Can you work these out from the model? Positions are in its coordinate system, mm. A direction names the side the tool comes from. Give positions to 0.01 mm unless a question says otherwise; leave off trailing zeros. Order: outer loops, then holes, each group sorted by start corner. A loop starts at its lowest first (then second) coordinate and runs counter-clockwise, first axis right, second up. Notation, with made-up numbers: (-35, 88.5) - (24, 88.5) arc R7 ccw to (24, 96.5) - close; hole circle Ø1 at (56, 83). An arc over 180 degrees is marked (long way). One line per question, with ' | ' between items.
Autodesk Inventor part; units mm, degrees
ref_plane "Work Plane1" through (4.68, 0, 0) normal (0, -0.866, 0.5) x (-1, 0, 0)
ref_plane "YZ Plane" through (0, 0, 0) normal (1, 0, 0) x (0, 1, 0)
ref_plane "XZ Plane" through (0, 0, 0) normal (0, 1, 0) x (-1, 0, 0)
sketch "Sketch1" plane through (0, 0, 0) normal (1, 0, 0) x (0, 1, 0)
  line L0 (-9.815, 0) -> (-4.9075, 8.5)
  line L1 (-4.9075, 8.5) -> (4.9075, 8.5)
  line L2 (4.9075, 8.5) -> (9.815, 0)
  line L3 (9.815, 0) -> (4.9075, -8.5)
  line L4 (4.9075, -8.5) -> (-4.9075, -8.5)
  line L5 (-4.9075, -8.5) -> (-9.815, 0)
  point P0 (0, 0)
  point P1 (0, 0)
  dimension "d0" = 19.6299
extrude "Body" add sketch "Sketch1" along normal blind 7.8
sketch "Sketch2" plane through (0, 0, 0) normal (0, 0, 1) x (1, 0, 0)
  line L0 (7.8, 8.5) -> (10.5, 8.5)
  line L1 (10.5, 8.5) -> (10.5, 5.8)
  line L2 (10.5, 5.8) -> (12.3, 5.8)
  arc A0 (18.1, 0) -> (12.3, 5.8) centre (12.3, 0) ccw
  line L3 (-3.8602, 0) -> (23.1615, 0)
  line L4 (0, -7.589) -> (0, 11.1815)
  line L5 (7.8, 0) -> (18.1, 0)
  line L6 (7.8, -4.9075) -> (7.8, 4.9075)
  line L7 (7.8, 0) -> (7.8, 8.5)
  point P0 (0, 0)
  dimension "d8" = 5.8
  dimension "d9" = 17
  dimension "d10" = 18.1
  dimension "d11" = 10.5
  dimension "d12" = 11.6
revolve "Cap" add sketch "Sketch2" angle 360 about axis through (7.8, 0, 0) along (1, 0, 0)
sketch "Sketch3" plane through (0, 0, 0) normal (-1, 0, 0) x (0, 0, 1)
  line L0 (0, -13.7409) -> (0, 13.7409)
  line L1 (-11.9, 0) -> (11.9, 0)
  point P0 (0, 0)
hole "Thread" at (0, 0, 0) direction (1, 0, 0) diameter 8.9175 depth 9.36 tip angle 118
sketch "Sketch4" plane through (0, 0, 0) normal (0, 0, 1) x (1, 0, 0)
  line L0 (0, 4.9075) -> (0, 9.815)
  line L1 (0, 9.815) -> (7.8, 9.815)
  line L2 (7.8, 4.9075) -> (7.8, 9.815)
  line L3 (-1.56, 0) -> (9.36, 0)
  line L4 (0, 8.5) -> (0.7592, 9.815)
  line L5 (7.8, 8.5) -> (7.0408, 9.815)
  dimension "d3" = 30
  dimension "d4" = 17
  dimension "d5" = 30
  dimension "d6" = 17
revolve "Chamfer1" cut sketch "Sketch4" angle 360 about axis through (-10, 0, 0) along (1, 0, 0)
chamfer "Chamfer2" distance 0.5413 angle 30 1 edges at (0, 0, -4.4587) measured on face at (0, 7.111, -0.1791)
ref_plane "Work Plane1" through (4.68, 0, 0) normal (0, -0.866, 0.5) x (-1, 0, 0)
equation "\"d0\" = 1.1547 * SW"
equation "\"d1\" = GEL"
equation "\"d8\" = KR"
equation "\"d9\" = SW"
equation "\"d10\" = KOH1"
equation "\"d11\" = SIH"
equation "\"d12\" = 2 * KR"
equation "\"d13\" = GEL"
equation "\"d14\" = 1.2 * GEL"
equation "\"d3\" = ANG1"
equation "\"d4\" = SW0"
equation "\"d5\" = ANG2"
equation "\"d6\" = SW"
equation "\"d17\" = -0.5 * GD1 + 0.5 * NND"
equation "\"d45\" = -0.5 * GD1 + 0.5 * NND"
equation "\"ANG1\" = 30deg"
equation "\"ANG2\" = 30deg"
equation "\"KOH1\" = 18.1"
equation "\"SW\" = 17"
equation "\"KR\" = 5.8"
equation "\"SIH\" = 10.5"
equation "\"GEL\" = 7.8"
equation "\"SW0\" = 17"
equation "\"GUL\" = 0.541266 * PTC"
equation "\"XKOH\" = 10.5"
equation "\"PTC\" = 1"
equation "\"TOA\" = 30deg"
equation "\"KOH0\" = 7.8"
equation "\"E0\" = 19.635"
equation "\"GAL\" = 0.541266 * PTC"
properties part number "CNS 4315 - M 10" material "Steel, Mild"
(1) Imagine slicing it at A-A (x = 4.25). List the corners of the cut face in (y, z) for me (1 decimal), and give its area (3 significant figures).
Answer below:
outline: (-9.8, 0) - (-4.9, -8.5) - (4.9, -8.5) - (9.8, 0) - (4.9, 8.5) - (-4.9, 8.5) - close; hole circle Ø8.9 at (0, 0) | area: 188 mm^2
(2) Imagine slicing it at C-C (x = 15). List the corners of the cut face in (y, z) for me.
Answer below:
outline: circle Ø10.27 at (0, 0)
(3) Will these pins go through, and if not, where does the flat tip stop? pin 1 (1 mm diameter, centred on y = 4, z = -6.5, fed in from +X); pin 2 (1 mm diameter, centred on y = 2, z = 1.5, fed in from +X); pin 3 (2 mm diameter, centred on x = 9, z = 2.5, fed in from +Y).
Answer below:
pin 1: x = 10.5 | pin 2: x = 17.74 | pin 3: y = 8.37
(4) If I drill on line 1 (Z direction, x = 6.25, y = 0); line 2 (X direction, y = -3.75, z = 7); line 3 (Z direction, x = 1.25, y = -2), over which ranges is the centre line in solid material (lowest first)?
Answer below:
line 1: -8.5 to -4.46, 4.46 to 8.5 | line 2: 0 to 10.5 | line 3: -8.5 to -3.99, 3.99 to 8.5
(5) On a 3-axis mill with a long thin cutter (end or side, diameter ignored), from which of +Z, -Z, +X, -X, +Y, -Y can I reach the whole of each face in a straight line? I mean faces 1 (the face through (4.9, 4.35, -0.97)), 2 (the face through (10.5, 2, -6)), 3 (the face through (3.845, -7.396, 4.19)). Say none if no direction works.
Answer below:
face 1: -X | face 2: +X | face 3: +Z, +X, -X, -Y
(6) Imagine slicing it at B-B (x = 9). List the corners of the cut face in (y, z) for me.
Answer below:
outline: circle Ø17 at (0, 0); hole circle Ø8.92 at (0, 0)
